CAD build for the part. Positions are in the model's coordinates, mm. Face numbers are marked on the shaded views. A direction names the side the tool comes from. Round coordinates to 2 decimals unless told otherwise and drop trailing zeros. Order: outer loops, then holes, each group sorted by start corner. A loop starts at its lowest first (then second) coordinate and runs counter-clockwise, first axis right, second up. Notation, with made-up numbers: (24.5, 61) - (54.5, 61) arc R35 ccw to (54.5, 94) - close; hole circle Ø10 at (-22.75, 25). An arc over 180 degrees is marked (long way). Use one line per item in the form item = value. Start each with the question number.
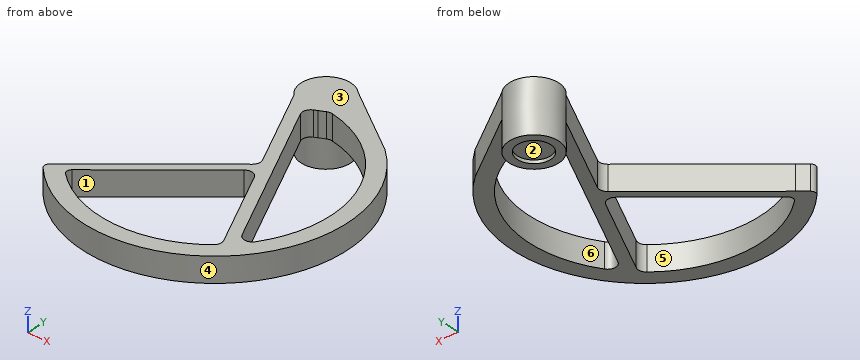
from build123d import *

# Parameters (mm, degrees)
EXTRUDE_1_DEPTH     = 15
CUT_EXTRUDE_START   = -15
CUT_EXTRUDE_1_DEPTH = 15
EXTRUDE_START       = 17
SKETCH_11_R         = 15
EXTRUDE_3_DEPTH     = 17
SKETCH_12_R         = 10.1
CUT_EXTRUDE_5_DEPTH = 2


with BuildPart() as part:
    # ｽｹｯﾁ4 → ﾎﾞｽ - 押し出し1 (new body)
    with BuildSketch(Plane.XY):
        with BuildLine():
            Line((-53.623111018, -124.995132678), (-58.940636287, -129.45706617))
            ThreePointArc((-58.940636287, -129.45706617), (-60.005384698, -131.552012131), (-59.233530865, -133.771635843))
            ThreePointArc((-59.233530865, -133.771635843), (57.362306223, -135.763481103), (52.076178918, -19.270504783))
            Line((52.076178918, -19.270504783), (10.606601718, 10.606601718))
            ThreePointArc((10.606601718, 10.606601718), (-10.606601718, 10.606601718), (-10.606601718, -10.606601718))
            Line((-10.606601718, -10.606601718), (14.536280154, -62.889638219))
            ThreePointArc((14.536280154, -62.889638219), (14.918089499, -66.109676181), (13.244185189, -68.886809092))
            Line((13.244185189, -68.886809092), (-53.623111018, -124.995132678))
        make_face()
        with BuildLine():
            Line((21.232400696, -76.813798404), (45.844843506, -127.993820346))
            ThreePointArc((45.844843506, -127.993820346), (46.221944165, -131.235480845), (44.518718993, -134.019289696))
            ThreePointArc((44.518718993, -134.019289696), (-2.231208213, -149.964431749), (-47.870174388, -131.072951785))
            ThreePointArc((-47.870174388, -131.072951785), (-48.817477846, -128.802229421), (-47.747678417, -126.586582094))
            Line((-47.747678417, -126.586582094), (13.511229465, -75.151532228))
            ThreePointArc((13.511229465, -75.151532228), (17.77869109, -74.092739753), (21.232400696, -76.813798404))
        make_face(mode=Mode.SUBTRACT)
    extrude(amount=EXTRUDE_1_DEPTH)

    # ｽｹｯﾁ6 → ｶｯﾄ - 押し出し1 (cut)
    with BuildSketch(Plane.XY.offset(15).offset(CUT_EXTRUDE_START)):
        with BuildLine():
            Line((49.189589797, -118.797265215), (2.201751786, -21.089020696))
            ThreePointArc((2.201751786, -21.089020696), (1.989274209, -17.268089629), (4.540836142, -14.416039025))
            Line((4.540836142, -14.416039025), (6.483415605, -13.48185369))
            Line((6.483415605, -13.48185369), (10.219658847, -11.685096486))
            ThreePointArc((10.219658847, -11.685096486), (11.747077013, -11.232198087), (13.339423466, -11.282754846))
            ThreePointArc((13.339423466, -11.282754846), (64.738421392, -53.37413296), (57.826055334, -119.448033215))
            ThreePointArc((57.826055334, -119.448033215), (53.319931874, -121.616182211), (49.189589797, -118.797265215))
        make_face()
    extrude(amount=CUT_EXTRUDE_1_DEPTH, mode=Mode.SUBTRACT)

    # ｽｹｯﾁ11 → ﾎﾞｽ - 押し出し3 (add)
    with BuildSketch(Plane(origin=(0, 0, 0), x_dir=(-1, 0, 0), z_dir=(0, 0, -1)).offset(EXTRUDE_START)):
        Circle(SKETCH_11_R)
    extrude(amount=-EXTRUDE_3_DEPTH)

    # ｽｹｯﾁ12 → ｶｯﾄ - 押し出し5 (cut)
    with BuildSketch(Plane(origin=(0, 0, -17), x_dir=(-1, 0, 0), z_dir=(0, 0, -1))):
        Circle(SKETCH_12_R)
    extrude(amount=-CUT_EXTRUDE_5_DEPTH, mode=Mode.SUBTRACT)


solid = part.part
(1) Slice it at D-D (x = 68). Give the cut face in (y, z).
(2) Wall check: line 1 (Y direction, x = 0, z = -16); line 2 (X direction, y = -85, z = 8.5); line 3 (Y direction, x = -4, z = 6). Give the ranges that are in metal, low to high. Write a range as [from, to].
(3) Which spindle directions (+Z, -Z, +X, -X, +Y, -Y) get a long thin tool onto all of the face, cutting with end or side? Do the marked faces 1 and 2. Say none if no direction does.
(4) Slice it at B-B (y = -40.5). Give the cut face in (x, z), and give its area (3 significant figures).
(5) Mould opens along X. For the marked faces 3, 4, 5 and 6 say: pulls with the +X half, pulls with the -X half, needs draft (parallel to the pull), parting line crosses it, or undercut.
(6) Flat gauge pins, fed straight in: P1, Ø3, axis at y = -16.5, z = 0, coming from the -X side; P2, Ø6, axis at x = 34, z = 3.5, coming from the +Y side. Where does each tip first touch, or does it go through?
(7) Slice it at C-C (y = -80). Give the cut face in (x, z), and give its area (3 significant figures).
(8) Slice it at A-A (z = 2). Give the cut face in (x, y), and give its area (3 significant figures).
Results list:
q1.outline = (-122.14, 0) - (-96.61, 0) - (-96.61, 15) - (-122.14, 15) - close; (-63.39, 0) - (-37.86, 0) - (-37.86, 15) - (-63.39, 15) - close
q2.line_1 = [-15, -10.1], [10.1, 15]
q2.line_2 = [-5.96, 1.78], [25.17, 32.94], [69.82, 79.84]
q2.line_3 = [-159.9, -149.89], [-89.85, -83.36], [-24.34, 14.46]
q3.face_1 = +Z, -Z
q3.face_2 = -Z
q4.outline = (3.77, 0) - (11.54, 0) - (11.54, 15) - (3.77, 15) - close; (57.79, 0) - (69.57, 0) - (69.57, 15) - (57.79, 15) - close
q4.area = 293 mm²
q5.face_3 = needs draft
q5.face_4 = parting line crosses it
q5.face_5 = undercut
q5.face_6 = undercut
q6.P1 = -8.49
q6.P2 = -4.09
q7.outline = (0, 0) - (7.74, 0) - (7.74, 15) - (0, 15) - close; (22.76, 0) - (30.53, 0) - (30.53, 15) - (22.76, 15) - close; (70, 0) - (80, 0) - (80, 15) - (70, 15) - close
q7.area = 383 mm²
q8.outline = (-59.23, -133.77) arc R80 ccw (long way) to (52.08, -19.27) - (10.61, 10.61) arc R15 ccw to (-10.61, -10.61) - (14.54, -62.89) arc R5 cw to (13.24, -68.89) - (-58.94, -129.46) arc R3 ccw to start; hole (-47.87, -131.07) arc R70 ccw to (44.52, -134.02) arc R5 ccw to (45.84, -127.99) - (21.23, -76.81) arc R5 ccw to (13.51, -75.15) - (-47.75, -126.59) arc R3 ccw to start; hole (2.2, -21.09) - (49.19, -118.8) arc R5 ccw to (57.83, -119.45) arc R70 ccw to (13.34, -11.28) arc R5 ccw to (10.22, -11.69) - (4.54, -14.42) arc R5 ccw to start
q8.area = 5,070 mm²
